Input: dimensioned drawing with shaded views. Units: mm. Origin: part minimum x, y, z. Coordinates: 2 decimals unless noted, no trailing zeros. Loops run counter-clockwise (first coordinate to the right, second up) from the corner with the lowest first, then second, coordinate; pieces in that order, holes last. Notation, with made-up numbers: (48.25, -8) -> (91.25, -8) arc R20 ccw to (91.25, 11) -> close; hole circle Ø1 at (32, -24). An arc over 180 degrees is marked (long way). Answer as CSV lines item,"result".
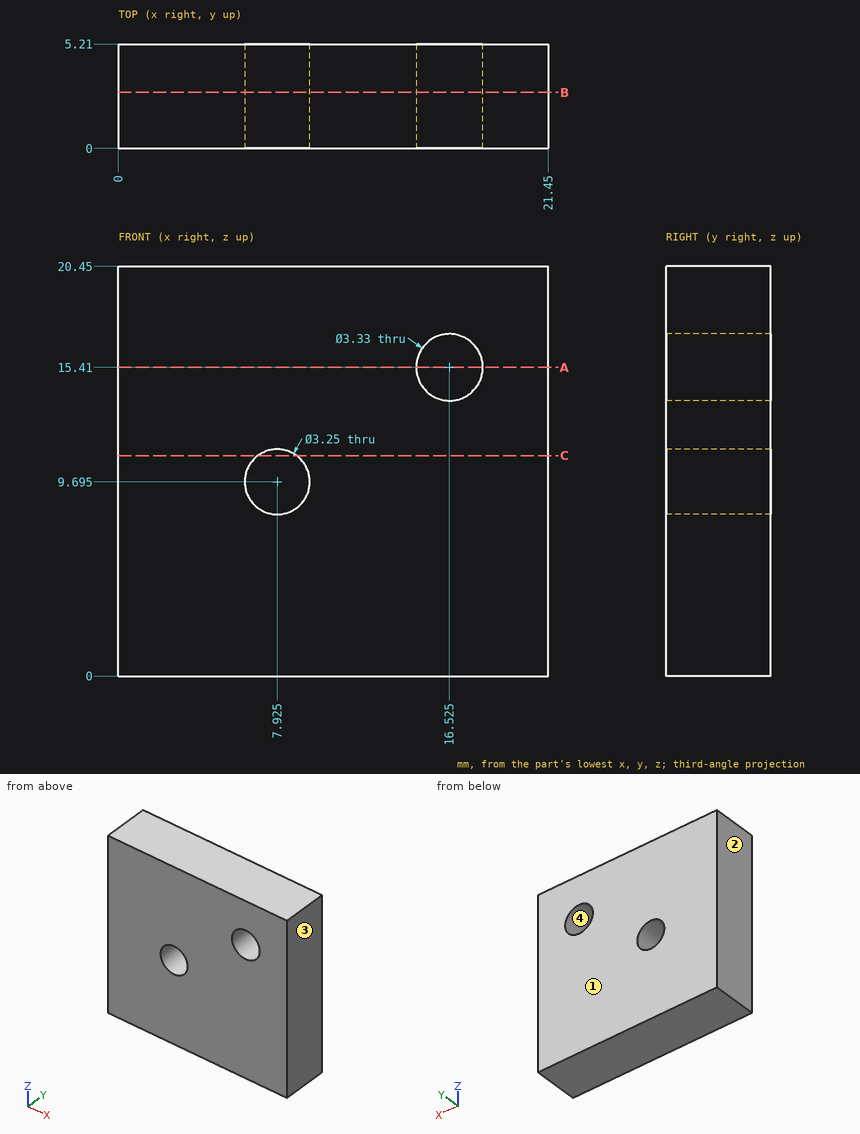
(1) Cut plane C-C (z = 11). Return the cut outline in (x, y).
Computed values:
outline,"(0, 0) -> (6.96, 0) -> (6.96, 5.21) -> (0, 5.21) -> close; (8.89, 0) -> (21.45, 0) -> (21.45, 5.21) -> (8.89, 5.21) -> close"
(2) Cut plane B-B (y = 2.8). Return the cut outline in (x, z) (3 decimals).
Computed values:
outline,"(0, 0) -> (21.45, 0) -> (21.45, 20.45) -> (0, 20.45) -> close; hole circle Ø3.25 at (7.925, 9.695); hole circle Ø3.33 at (16.525, 15.41)"
(3) Draft query along X for the marked faces 1, 2, 3 and 4. Return one class per face: released by +X, released by -X, zero draft, split by the parting line, or undercut.
Computed values:
face 1,"zero draft"
face 2,"released by -X"
face 3,"released by +X"
face 4,"undercut"
(4) Material intervals for L1, parallel to Z at x = 8, y = 1.4; L2, parallel to X at y = 3.9, z = 10.75; L3, parallel to Z at x = 9.25, y = 1.5, sorted ascending. Write a range as [from, to].
Computed values:
L1,"[0, 8.07], [11.32, 20.45]"
L2,"[0, 6.69], [9.16, 21.45]"
L3,"[0, 8.75], [10.64, 20.45]"
(5) Cut plane A-A (z = 15.41). Return the cut outline in (x, y), then the cut area to 3 significant figures.
Computed values:
outline,"(0, 0) -> (14.86, 0) -> (14.86, 5.21) -> (0, 5.21) -> close; (18.19, 0) -> (21.45, 0) -> (21.45, 5.21) -> (18.19, 5.21) -> close"
area,"94.4 mm^2"
